Check sheet for the drawn part. Datum: minimum x, y, z corner. Units: mm. Round coordinates to 2 decimals unless told otherwise and drop trailing zeros. Loops run counter-clockwise (first coordinate to the right, second up) from the corner with the lowest first, then second, coordinate; pieces in that order, holes last. Notation, with made-up numbers: (53.5, 9.25) -> (85.5, 9.25) arc R26 cw to (85.5, 41.25) -> close; hole circle Ø10 at (-15, 26.25). An arc over 180 degrees is marked (long way). Return JSON: item names as keys, results as strings.
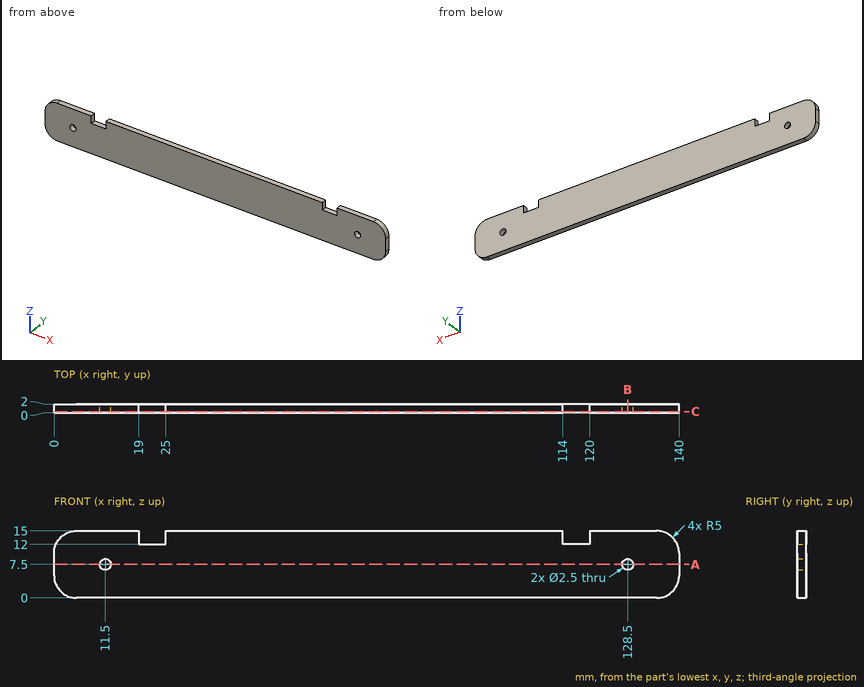
Q1. Go/stop test with flat-tipped pins: pin 1 (0.6 mm diameter, centred on x = 21.5, y = 0.5, fed in from +Z); pin 2 (1 mm diameter, centred on y = 0.5, z = 11, fed in from +X); pin 3 (0.6 mm diameter, centred on y = 1, z = 14, fed in from +X). Record where each tip stops, or that it passes through.
Results list:
{"pin 1": "z = 12", "pin 2": "x = 139.97", "pin 3": "x = 138.36"}
Q2. Section check C-C (y = 0.3). Record the boundary of the cut face in (x, z), then the cut area to 3 significant figures.
Results list:
{"outline": "(0, 5) arc R5 ccw to (5, 0) -> (135, 0) arc R5 ccw to (140, 5) -> (140, 10) arc R5 ccw to (135, 15) -> (120, 15) -> (120, 12) -> (114, 12) -> (114, 15) -> (25, 15) -> (25, 12) -> (19, 12) -> (19, 15) -> (5, 15) arc R5 ccw to (0, 10) -> close; hole circle Ø2.5 at (11.5, 7.5); hole circle Ø2.5 at (128.5, 7.5)", "area": "2,030 mm^2"}
Q3. Section check B-B (x = 128.5). Record the boundary of the cut face in (y, z), then the cut area to 3 significant figures.
Results list:
{"outline": "(0, 0) -> (2, 0) -> (2, 6.25) -> (0, 6.25) -> close; (0, 8.75) -> (2, 8.75) -> (2, 15) -> (0, 15) -> close", "area": "25.0 mm^2"}
Q4. Material ranges on line 1 (X direction, y = 1.15, z = 7.5); line 2 (Z direction, x = 11.5, y = 1.2); line 3 (X direction, y = 1.4, z = 12.25), recorded low to high.
Results list:
{"line 1": "0 to 10.25, 12.75 to 127.25, 129.75 to 140", "line 2": "0 to 6.25, 8.75 to 15", "line 3": "0.53 to 19, 25 to 114, 120 to 139.47"}
Q5. Section check A-A (z = 7.5). Record the boundary of the cut face in (x, y), then the cut area to 3 significant figures.
Results list:
{"outline": "(0, 0) -> (10.25, 0) -> (10.25, 2) -> (0, 2) -> close; (12.75, 0) -> (127.25, 0) -> (127.25, 2) -> (12.75, 2) -> close; (129.75, 0) -> (140, 0) -> (140, 2) -> (129.75, 2) -> close", "area": "270 mm^2"}
